Autodesk Inventor part; units mm, degrees
ref_plane "YZ Plane" through (0, 0, 0) normal (1, 0, 0) x (0, 1, 0)
ref_plane "XZ Plane" through (0, 0, 0) normal (0, 1, 0) x (-1, 0, 0)
ref_plane "XY Plane" through (0, 0, 0) normal (0, 0, 1) x (1, 0, 0)
sketch "Sketch1" plane through (0, 0, 0) normal (0, 1, 0) x (-1, 0, 0)
  line L0 (93, -25) -> (-93, -25)
  line L1 (-93, -25) -> (-93, 25)
  line L2 (-93, 25) -> (93, 25)
  line L3 (93, 25) -> (93, -25)
  line L4 (93, -25) -> (-93, 25) construction
  line L5 (-93, -25) -> (93, 25) construction
  line L6 (73, -11) -> (-47, -11)
  line L7 (-47, -11) -> (-47, 8)
  line L8 (-47, 8) -> (73, 8)
  line L9 (73, 8) -> (73, -11)
  point P0 (0, 0)
  dimension "d0" = 186
  dimension "d1" = 50
  dimension "d2" = 17
  dimension "d3" = 36
  dimension "d4" = 120
  dimension "d5" = 20
extrude "Extrusion1" add sketch "Sketch1" along normal blind 3
chamfer "Chamfer3" distance 3 angle 45 1 edges at (-93, 0, 0) measured on face at (-93, 1, -8.3333)
chamfer "Chamfer4" distance 3 angle 45 1 edges at (93, 0, 0) measured on face at (93, 1, 8.3333)
properties part number "Front Wall"
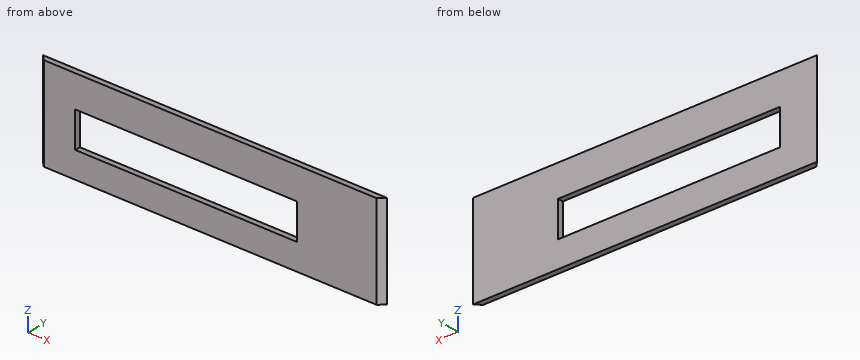
Here's how the part is built. I have some questions about the finished solid (model axes, mm). Round coordinates to 2 decimals unless told otherwise and drop trailing zeros. Loops run counter-clockwise (first coordinate to the right, second up) from the corner with the lowest first, then second, coordinate; pieces in that order, holes last. Notation, with made-up numbers: (10.5, 63) -> (54.5, 63) arc R20 cw to (54.5, 98) -> close; hole circle Ø11 at (14, 36.25). An arc over 180 degrees is marked (long way). Write each question's results on one line, items separated by ' | '.
(1) For P1, Ø0.9, axis at y = 2, z = 0.5, coming from the -X side; P2, Ø0.9, axis at y = 1.5, z = 1.5, coming from the +X side, each with a flat end and sliding along its axis, tell me the tip position at first contact or that it passes through.
Worked answers:
P1: x = -92.45 | P2: x = 91.95
(2) If we section it at B-B, the plane x = -41.5: List the corners of the cut face in (y, z) for me, then the cut area to 3 significant figures.
Worked answers:
outline: (0, -25) -> (3, -25) -> (3, -11) -> (0, -11) -> close; (0, 8) -> (3, 8) -> (3, 25) -> (0, 25) -> close | area: 93.0 mm2
(3) If we section it at C-C, the plane y = 1.1: List the corners of the cut face in (x, z) for me, then the cut area to 3 significant figures.
Worked answers:
outline: (-91.1, -25) -> (91.1, -25) -> (91.1, 25) -> (-91.1, 25) -> close; hole (-73, -11) -> (47, -11) -> (47, 8) -> (-73, 8) -> close | area: 6,830 mm2
(4) If I drill on L1, parallel to Z at x = 14, y = 1.9; L2, parallel to X at y = 2.5, z = -5; L3, parallel to X at y = 2.4, z = 22, over which ranges is the centre line in solid material (lowest first)?
Worked answers:
L1: -25 to -11, 8 to 25 | L2: -92.5 to -73, 47 to 92.5 | L3: -92.4 to 92.4
